Build history of the part. All positions in model axes, mm. A direction names the side the tool comes from. Round coordinates to 2 decimals unless told otherwise and drop trailing zeros. Write each loop counter-clockwise with the first axis right and the second up, starting at its lowest first coordinate (ties: lowest second). Pieces come first, ordered by that corner, then holes. Notation, with made-up numbers: (-20, 65.5) - (-5, 65.5) arc R29 ccw to (-5, 97.5) - close; hole circle Ø8 at (72, 60.5). An arc over 180 degrees is marked (long way). Write each question's results on one line, items separated by ' | '.
from build123d import *

# Parameters (mm, degrees)
SKETCH_1_W          = 280
SKETCH_1_H          = 63
SKETCH_1_R          = 2
EXTRUDE_1_DEPTH     = 3
CUT_EXTRUDE_1_DEPTH = 3
SKETCH_3_W          = 200
SKETCH_3_H          = 63
CUT_EXTRUDE_2_DEPTH = 10
CUT_EXTRUDE_3_DEPTH = 10
CUT_EXTRUDE_4_DEPTH = 10
FILLET_1_R          = 2


with BuildPart() as part:
    # 草图1 → 凸台-拉伸1 (new body)
    with BuildSketch(Plane(origin=(0, 0, 0), x_dir=(1, 0, 0), z_dir=(0, 1, 0))):
        Rectangle(SKETCH_1_W, SKETCH_1_H)
        with Locations(Location((-65, 26.5, 0), (0, 0, 270))):
            Circle(SKETCH_1_R, mode=Mode.SUBTRACT)
        with Locations(Location((-65, -26.5, 0), (0, 0, 270))):
            Circle(SKETCH_1_R, mode=Mode.SUBTRACT)
        with Locations(Location((65, -26.5, 0), (0, 0, 90))):
            Circle(SKETCH_1_R, mode=Mode.SUBTRACT)
        with Locations(Location((65, 26.5, 0), (0, 0, 90))):
            Circle(SKETCH_1_R, mode=Mode.SUBTRACT)
    extrude(amount=EXTRUDE_1_DEPTH)

    # 草图2 → 切除-拉伸1 (cut)
    with BuildSketch(Plane(origin=(0, 3, 0), x_dir=(1, 0, 0), z_dir=(0, 1, 0))):
        Polygon((-140, 18.5), (-140, -31.5), (-90, -31.5), align=None)
        Polygon((90, -31.5), (140, 18.5), (140, -31.5), align=None)
    extrude(amount=-CUT_EXTRUDE_1_DEPTH, mode=Mode.SUBTRACT)

    # 草图3 → 切除-拉伸2 (cut)
    with BuildSketch(Plane(origin=(0, 3, 0), x_dir=(1, 0, 0), z_dir=(0, 1, 0))):
        with Locations((40, 0)):
            Rectangle(SKETCH_3_W, SKETCH_3_H)
    extrude(amount=-CUT_EXTRUDE_2_DEPTH, mode=Mode.SUBTRACT)

    # 草图4 → 切除-拉伸3 (cut)
    with BuildSketch(Plane(origin=(0, 3, 0), x_dir=(1, 0, 0), z_dir=(0, 1, 0))):
        Polygon((-115, 31.5), (-110, 26.5), (-75, 26.5), (-70, 31.5), align=None)
    extrude(amount=-CUT_EXTRUDE_3_DEPTH, mode=Mode.SUBTRACT)

    # 草图5 → 切除-拉伸4 (cut)
    with BuildSketch(Plane(origin=(0, 3, 0), x_dir=(1, 0, 0), z_dir=(0, 1, 0))):
        Polygon((-127.857864376, 20.5), (-70, 20.5), (-70, -19.5), (-87.857864376, -19.5), align=None)
    extrude(amount=-CUT_EXTRUDE_4_DEPTH, mode=Mode.SUBTRACT)

    # 圆角1
    fillet_1_edges = [part.edges().sort_by_distance(p)[0] for p in [
        (-70, 1.5, -20.5),
        (-70, 1.5, 19.5),
        (-87.857864376, 1.5, 19.5),
        (-127.857864376, 1.5, -20.5),
    ]]
    fillet(fillet_1_edges, radius=FILLET_1_R)


solid = part.part
(1) Flat gauge pins, fed straight in: pin 1 Ø6.5 at (x, z) = (-65, -26.5) entering from -Y; pin 2 Ø0.9 at (y, z) = (2, 7) entering from -X; pin 3 Ø0.9 at (x, y) = (-95, 1) entering from +Z; pin 4 Ø1.5 at (y, z) = (1.5, 25) entering from -X. Where does each tip first touch, or does it go through?
Worked answers:
pin 1: stops at y = 0 | pin 2: stops at x = -114.95 | pin 3: stops at z = 26.95 | pin 4: stops at x = -97.25
(2) Slice it at A-A, the plane z = 26.5. Write the cut outline in (x, y), and give its area (3 significant figures).
Worked answers:
outline: (-95, 0) - (-67, 0) - (-67, 3) - (-95, 3) - close; (-63, 0) - (-60, 0) - (-60, 3) - (-63, 3) - close | area: 93.0 mm2
(3) Two-plate mould, pull along X, no slides. Class faces 1 (the flat face through (-140, 1, -25)), 2 (the flat face through (-109, 3, 0)), 3 (the flat face through (-79, 2, 19.5)): released by +X, released by -X, zero draft, split by the parting line, or undercut.
Worked answers:
face 1: released by -X | face 2: zero draft | face 3: undercut
(4) Slice it at B-B, the plane x = -84.5. Write the cut outline in (y, z), and give its area (3 significant figures).
Worked answers:
outline: (0, -26.5) - (3, -26.5) - (3, -20.5) - (0, -20.5) - close; (0, 19.5) - (3, 19.5) - (3, 31.5) - (0, 31.5) - close | area: 54.0 mm2
(5) Drill centre lines: probe 1 along Z at (x, y) = (-79.5, 2.8); probe 2 along Z at (x, y) = (-89, 2.65); probe 3 along X at (y, z) = (0.95, -7.5). Where is each one in solid material? Low to high. Write a range as [from, to].
Worked answers:
probe 1: z = [-26.5, -20.5], [19.5, 31.5] | probe 2: z = [-26.5, -20.5], [18.36, 31.5] | probe 3: x = [-129, -114.86], [-70, -60]
(6) Tool access for faces 4 (the cylindrical face through (-70.57, 1.48, -19.9)), 5 (the flat face through (-112.5, 1.5, -29)), 6 (the flat face through (-114.65, 1.52, 6.85)): list every direction of +Z, -Z, +X, -X, +Y, -Y with a clear straight run to the whole face (end or side of a thin tool).
Worked answers:
face 4: +Y, -Y | face 5: -Z, +Y, -Y | face 6: +Z, -X, +Y, -Y
(7) Slice it at C-C, the plane y = 2.5. Write the cut outline in (x, z).
Worked answers:
outline: (-140, -31.5) - (-115, -31.5) - (-110, -26.5) - (-75, -26.5) - (-70, -31.5) - (-60, -31.5) - (-60, 31.5) - (-90, 31.5) - (-140, -18.5) - close; hole (-124.44, -17.09) arc R2 ccw to (-123.03, -20.5) - (-72, -20.5) arc R2 ccw to (-70, -18.5) - (-70, 17.5) arc R2 ccw to (-72, 19.5) - (-87.03, 19.5) arc R2 ccw to (-88.44, 18.91) - close; hole circle Ø4 at (-65, -26.5); hole circle Ø4 at (-65, 26.5)
(8) Slice it at D-D, the plane x = -65. Write the cut outline in (y, z).
Worked answers:
outline: (0, -31.5) - (3, -31.5) - (3, -28.5) - (0, -28.5) - close; (0, -24.5) - (3, -24.5) - (3, 24.5) - (0, 24.5) - close; (0, 28.5) - (3, 28.5) - (3, 31.5) - (0, 31.5) - close
